Geometry: final body of the model. Coordinates: model frame, mm. Face numbers are marked on the shaded views. A direction names the side the tool comes from. Coordinates: 2 decimals unless noted, no trailing zeros. Loops run counter-clockwise (first coordinate to the right, second up) from the corner with the lowest first, then second, coordinate; pieces in that order, holes last. Notation, with made-up numbers: M -5.5,55.25 L 24.5,55.25 A18 ccw 24.5,73.25 Z; hole C -9,0 d11. An arc over 180 degrees is marked long. Write each question's results on one line, items separated by ' | '. Start each with the question number.
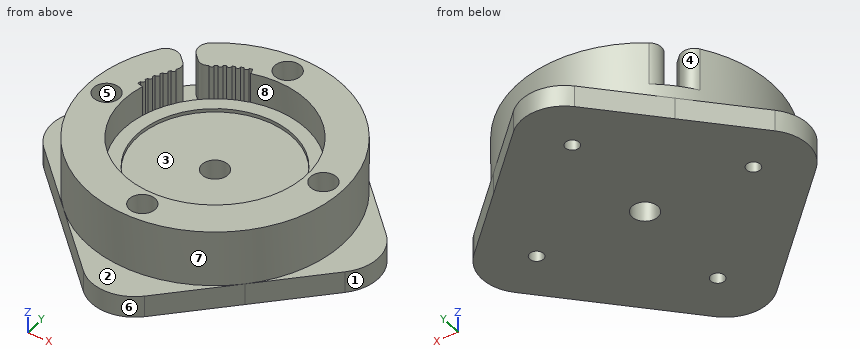
from build123d import *

# Parameters (mm, degrees)
SKETCH_01_W               = 8.999999864
SKETCH_01_H               = 30.367248618
CUT_EXTRUDE_01_DEPTH      = 4.499999932
CUT_EXTRUDE_01_DEPTH_BACK = 4.499999932
SKETCH_433_W              = 8.999999864
SKETCH_433_H              = 0.009842519
SKETCH_5_R                = 36.024182257
SKETCH_5_R_2              = 29.54824863
CUT_EXTRUDE_2_DEPTH       = 10
EXTRUDE_START             = 9
SKETCH_6_R                = 29.54824863
EXTRUDE_1_DEPTH           = 9
SKETCH_7_R                = 21.1
CUT_EXTRUDE_3_DEPTH       = 7
SKETCH_8_R                = 1.6
CUT_EXTRUDE_4_DEPTH       = 34
SKETCH_9_R                = 3
CUT_EXTRUDE_5_DEPTH       = 34
SKETCH_10_R               = 18
CUT_EXTRUDE_6_DEPTH       = 0.8
SKETCH_12_R               = 3
CUT_EXTRUDE_8_DEPTH       = 5
EXTRUDE_2_DEPTH           = 5
CUT_EXTRUDE_9_DEPTH       = 10
FILLET_1_R                = 3


with BuildPart() as part:
    # Sketch 01 → 同步带轮01 (revolve)
    with BuildSketch(Plane(origin=(0, 0, 0), x_dir=(0, 0, -1), z_dir=(1, 0, 0)), mode=Mode.PRIVATE) as revolve_01_sk:
        with Locations((0, 15.183624309)):
            Rectangle(SKETCH_01_W, SKETCH_01_H)
    revolve(revolve_01_sk.sketch.rotate(Axis((0, 0, 0), (0, 0, -1)), 90), axis=Axis((0, 0, 0), (0, 0, -1)))

    # Sketch 01 2 → 齿拉伸切除同步带轮01 (cut, two sides: drawn at the far end of the back side and taken through both)
    with BuildSketch(Plane.XY.offset(-CUT_EXTRUDE_01_DEPTH_BACK)):
        with BuildLine():
            Line((-0.813748126, 30.356343696), (0, 32.907248579))
            Line((0, 32.907248579), (0.813748126, 30.356343696))
            ThreePointArc((0.813748126, 30.356343696), (0.662957144, 30.297406109), (0.599999991, 30.148248621))
            ThreePointArc((0.599999991, 30.148248621), (0, 29.54824863), (-0.599999991, 30.148248621))
            ThreePointArc((-0.599999991, 30.148248621), (-0.662957144, 30.297406109), (-0.813748126, 30.356343696))
        make_face()
    extrude(amount=CUT_EXTRUDE_01_DEPTH + CUT_EXTRUDE_01_DEPTH_BACK, mode=Mode.SUBTRACT)

    # Sketch 433 → Cut-Revolve 471 (revolve, cut)
    with BuildSketch(Plane(origin=(0, 0, 0), x_dir=(0, 0, -1), z_dir=(1, 0, 0)), mode=Mode.PRIVATE) as cut_revolve_471_sk:
        with Locations((0, 0.00492126)):
            Rectangle(SKETCH_433_W, SKETCH_433_H)
    revolve(cut_revolve_471_sk.sketch.rotate(Axis((0, 0, 0), (0, 0, -1)), 90), axis=Axis((0, 0, 0), (0, 0, -1)), mode=Mode.SUBTRACT)

    # 草图5 → 切除-拉伸2 (cut)
    with BuildSketch(Plane(origin=(0, 0, -4.499999932), x_dir=(-1, 0, 0), z_dir=(0, 0, -1))):
        Circle(SKETCH_5_R)
        Circle(SKETCH_5_R_2, mode=Mode.SUBTRACT)
    extrude(amount=-CUT_EXTRUDE_2_DEPTH, mode=Mode.SUBTRACT)

    # 草图6 → 凸台-拉伸1 (add)
    with BuildSketch(Plane(origin=(0, 0, -4.499999932), x_dir=(-1, 0, 0), z_dir=(0, 0, -1)).offset(EXTRUDE_START)):
        Circle(SKETCH_6_R)
    extrude(amount=-EXTRUDE_1_DEPTH)

    # 草图7 → 切除-拉伸3 (cut)
    with BuildSketch(Plane.XY.offset(4.499999932)):
        Circle(SKETCH_7_R)
    extrude(amount=-CUT_EXTRUDE_3_DEPTH, mode=Mode.SUBTRACT)

    # 草图8 → 切除-拉伸4 (cut)
    with BuildSketch(Plane.XY.offset(4.499999932)):
        with Locations((0, 25)):
            Circle(SKETCH_8_R)
        with Locations((25, 0)):
            Circle(SKETCH_8_R)
        with Locations((0, -25)):
            Circle(SKETCH_8_R)
        with Locations((-25, 0)):
            Circle(SKETCH_8_R)
    extrude(amount=-CUT_EXTRUDE_4_DEPTH, mode=Mode.SUBTRACT)

    # 草图9 → 切除-拉伸5 (cut)
    with BuildSketch(Plane.XY.offset(-2.500000068)):
        Circle(SKETCH_9_R)
    extrude(amount=-CUT_EXTRUDE_5_DEPTH, mode=Mode.SUBTRACT)

    # 草图10 → 切除-拉伸6 (cut)
    with BuildSketch(Plane.XY.offset(-2.500000068)):
        Circle(SKETCH_10_R)
    extrude(amount=-CUT_EXTRUDE_6_DEPTH, mode=Mode.SUBTRACT)

    # 草图12 → 切除-拉伸8 (cut)
    with BuildSketch(Plane.XY.offset(4.499999932)):
        with Locations((0, -25)):
            Circle(SKETCH_12_R)
        with Locations((-25, 0)):
            Circle(SKETCH_12_R)
        with Locations((0, 25)):
            Circle(SKETCH_12_R)
        with Locations((25, 0)):
            Circle(SKETCH_12_R)
    extrude(amount=-CUT_EXTRUDE_8_DEPTH, mode=Mode.SUBTRACT)

    # 草图13 → 凸台-拉伸2 (add)
    with BuildSketch(Plane(origin=(0, 0, -13.499999932), x_dir=(-1, 0, 0), z_dir=(0, 0, -1))):
        with BuildLine():
            Line((-7.071067812, 34.716466145), (-20.893766978, 20.893766978))
            ThreePointArc((-20.893766978, 20.893766978), (0, 29.54824863), (20.893766978, 20.893766978))
            Line((20.893766978, 20.893766978), (7.071067812, 34.716466145))
            ThreePointArc((7.071067812, 34.716466145), (0, 37.645398333), (-7.071067812, 34.716466145))
        make_face()
        with BuildLine():
            Line((-34.716466145, -7.071067812), (-20.893766978, -20.893766978))
            ThreePointArc((-20.893766978, -20.893766978), (-29.54824863, 0), (-20.893766978, 20.893766978))
            Line((-20.893766978, 20.893766978), (-34.716466145, 7.071067812))
            ThreePointArc((-34.716466145, 7.071067812), (-37.645398333, 0), (-34.716466145, -7.071067812))
        make_face()
        with BuildLine():
            ThreePointArc((-7.071067812, -34.716466145), (0, -37.645398333), (7.071067812, -34.716466145))
            Line((7.071067812, -34.716466145), (20.893766881, -20.893767076))
            ThreePointArc((20.893766881, -20.893767076), (-6.9e-08, -29.54824863), (-20.893766978, -20.893766978))
            Line((-20.893766978, -20.893766978), (-7.071067812, -34.716466145))
        make_face()
        with BuildLine():
            ThreePointArc((29.54824863, 0), (27.299022104, -11.30762527), (20.893766881, -20.893767076))
            Line((20.893766881, -20.893767076), (34.716466145, -7.071067812))
            ThreePointArc((34.716466145, -7.071067812), (37.645398333, 0), (34.716466145, 7.071067812))
            Line((34.716466145, 7.071067812), (20.893766978, 20.893766978))
            ThreePointArc((20.893766978, 20.893766978), (27.299022131, 11.307625206), (29.54824863, 0))
        make_face()
    extrude(amount=-EXTRUDE_2_DEPTH)

    # 草图14 → 切除-拉伸9 (cut)
    with BuildSketch(Plane.XY.offset(4.499999932)):
        with BuildLine():
            Line((-21.733331092, 5.823428515), (-20.381034935, 5.461081852))
            ThreePointArc((-20.381034935, 5.461081852), (-14.919953083, 14.919953083), (-5.461081852, 20.381034935))
            Line((-5.461081852, 20.381034935), (-5.763920314, 21.511243463))
            ThreePointArc((-5.763920314, 21.511243463), (-5.832067357, 21.608637877), (-5.875298538, 21.719366176))
            ThreePointArc((-5.875298538, 21.719366176), (-6.212606996, 21.625298017), (-6.548410612, 21.525991695))
            ThreePointArc((-6.548410612, 21.525991695), (-6.869005795, 20.900161707), (-7.498359319, 21.213783433))
            ThreePointArc((-7.498359319, 21.213783433), (-7.827602785, 21.094516696), (-8.154950219, 20.970140365))
            ThreePointArc((-8.154950219, 20.970140365), (-8.427379648, 20.321891454), (-9.078615536, 20.5871013))
            ThreePointArc((-9.078615536, 20.5871013), (-9.397914516, 20.443316823), (-9.714937098, 20.294580488))
            ThreePointArc((-9.714937098, 20.294580488), (-9.937645604, 19.627613198), (-10.60704626, 19.842897209))
            ThreePointArc((-10.60704626, 19.842897209), (-10.914578029, 19.675415789), (-11.219466026, 19.503168514))
            ThreePointArc((-11.219466026, 19.503168514), (-11.391182272, 18.821290244), (-12.074926408, 18.985419464))
            ThreePointArc((-12.074926408, 18.985419464), (-12.368935412, 18.795197173), (-12.659948365, 18.600422237))
            ThreePointArc((-12.659948365, 18.600422237), (-12.779692104, 17.907525505), (-13.47387655, 18.019563))
            ThreePointArc((-13.47387655, 18.019563), (-14.814779333, 17.626436866), (-16.085768028, 18.207088371))
            Line((-16.085768028, 18.207088371), (-19.806167535, 21.927487879))
            ThreePointArc((-19.806167535, 21.927487879), (-20.893766978, 20.893766978), (-21.927487879, 19.806167535))
            Line((-21.927487879, 19.806167535), (-18.207088371, 16.085768028))
            ThreePointArc((-18.207088371, 16.085768028), (-17.626436866, 14.814779333), (-18.019563, 13.47387655))
            ThreePointArc((-18.019563, 13.47387655), (-17.907525505, 12.779692104), (-18.600422237, 12.659948365))
            ThreePointArc((-18.600422237, 12.659948365), (-18.795197173, 12.368935412), (-18.985419464, 12.074926408))
            ThreePointArc((-18.985419464, 12.074926408), (-18.821290244, 11.391182272), (-19.503168514, 11.219466026))
            ThreePointArc((-19.503168514, 11.219466026), (-19.675415789, 10.914578029), (-19.842897209, 10.60704626))
            ThreePointArc((-19.842897209, 10.60704626), (-19.627613198, 9.937645604), (-20.294580488, 9.714937098))
            ThreePointArc((-20.294580488, 9.714937098), (-20.443316823, 9.397914516), (-20.5871013, 9.078615536))
            ThreePointArc((-20.5871013, 9.078615536), (-20.321891454, 8.427379648), (-20.970140365, 8.154950219))
            ThreePointArc((-20.970140365, 8.154950219), (-21.094516696, 7.827602785), (-21.213783433, 7.498359319))
            ThreePointArc((-21.213783433, 7.498359319), (-20.900161707, 6.869005795), (-21.525991695, 6.548410612))
            ThreePointArc((-21.525991695, 6.548410612), (-21.63269867, 6.186788202), (-21.733331092, 5.823428515))
        make_face()
    extrude(amount=-CUT_EXTRUDE_9_DEPTH, mode=Mode.SUBTRACT)

    # 圆角1
    fillet_1_edges = [part.edges().sort_by_distance(p)[0] for p in [
        (-19.806167535, 21.927487879, -0.500000068),
        (-21.927487879, 19.806167535, -0.500000068),
    ]]
    fillet(fillet_1_edges, radius=FILLET_1_R)


solid = part.part
Item 1: Section C-C, the plane y = 0. Count the separate pieces of the cut face and the enclosed holes in it, plus the area to 3 significant figures.
Item 2: Pull-direction query (Y, two-part tool) for the marked faces 5, 6, 7 and 8; classes: released by +Y, released by -Y, zero draft, split by the parting line, or undercut.
Item 3: Set-up query: the marked faces 1, 2, 3 and 4. Return all of +Z, -Z, +X, -X, +Y, -Y with unobstructed straight access to the full face (end or side cutting, diameter ignored); none if empty.
Item 4: Section B-B, the plane z = -12. Return loops of the section in (x, y).
Item 5: Ray query, L1, parallel to Z at x = 2, y = -23; L2, parallel to Y at x = 25, z = -10.5; L3, parallel to Y at x = -8, z = 3. Return the intervals inside material, ascending. Write a range as [from, to].
Item 6: Contact query for flat-ended pins moving along their axis: P1, Ø6.5, axis at x = 1.5, y = 24, coming from the +Z side; P2, Ø1.8, axis at x = 24.5, y = 0, coming from the +Z side; P3, Ø2, axis at y = -16.5, z = -2.5, coming from the +X side; P4, Ø4, axis at x = 25, y = 0, coming from the +Z side. Output: stop coordinate, or through.
Item 7: Section A-A, the plane x = 25. Return loops of the section in (y, z).
Solutions:
1) separate pieces: 4 | enclosed holes: 0 | area: 616 mm²
2) face 5: undercut | face 6: released by -Y | face 7: split by the parting line | face 8: undercut
3) face 1: +Z, -Z, +X | face 2: +Z, -Y | face 3: +Z | face 4: +Z, +Y
4) outline: M -34.72,-7.07 L -7.07,-34.72 A10 ccw 7.07,-34.72 L 34.72,-7.07 A10 ccw 34.72,7.07 L 7.07,34.72 A10 ccw -7.07,34.72 L -34.72,7.07 A10 ccw Z; hole C -25,0 d3.2; hole C 0,0 d6; hole C 0,-25 d3.2; hole C 0,25 d3.2; hole C 25,0 d3.2
5) L1: z = [-13.5, -0.5] | L2: y = [-16.79, -1.6], [1.6, 16.79] | L3: y = [-28.44, -19.52], [21.03, 28.44]
6) P1: stops at z = 4.5 | P2: passes through | P3: stops at x = 25.16 | P4: stops at z = -0.5
7) outline: M -16.79,-13.5 L -1.6,-13.5 L -1.6,-0.5 L -3,-0.5 L -3,4.5 L -15.75,4.5 L -15.75,-8.5 L -16.79,-8.5 Z; M 1.6,-13.5 L 16.79,-13.5 L 16.79,-8.5 L 15.75,-8.5 L 15.75,4.5 L 3,4.5 L 3,-0.5 L 1.6,-0.5 Z
